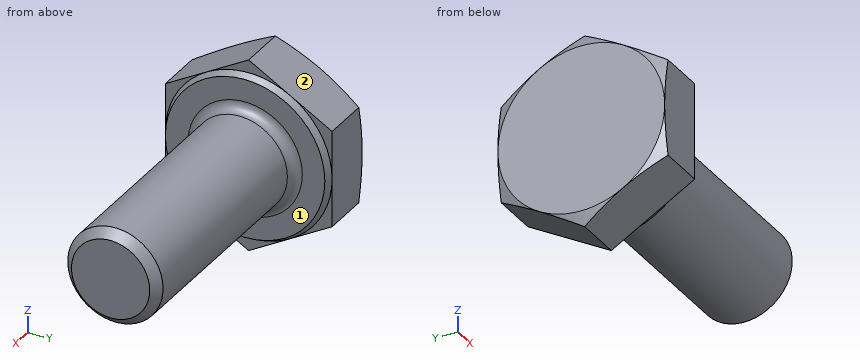
Autodesk Inventor part; units mm, degrees
ref_plane "Work Plane1" through (0, 10.5, -6.0622) normal (0, 0.5, 0.8660254) x (-1, 0, 0)
ref_plane "YZ Plane" through (0, 0, 0) normal (1, 0, 0) x (0, 1, 0)
ref_plane "XZ Plane" through (0, 0, 0) normal (0, 1, 0) x (-1, 0, 0)
sketch "草图4" plane through (0, 0, 0) normal (0, 0, 1) x (1, 0, 0)
  line L0 (0, 0) -> (0, 10.5)
  line L1 (0, 10.5) -> (0.8, 10.0381)
  line L2 (0.8, 10.0381) -> (0.8, 0)
  line L3 (0.8, 0) -> (0, 0)
  line L4 (0, 0) -> (10.723, 0)
  line L5 (0.8, 0) -> (30.8, 0)
  line L6 (30.8, 0) -> (30.8, 6)
  line L7 (30.8, 6) -> (0.8, 6)
  line L8 (0.8, 6) -> (0.8, 0)
  dimension "INC" = 0.8
  dimension "d22" = 60
  dimension "L" = 30
  dimension "D" = 12
  dimension "INS" = 21
revolve "Revolution3" add sketch "草图4" angle 360 about axis through (0, 0, 0) along (1, 0, 0)
sketch "草图5" plane through (0, 0, 0) normal (-1, 0, 0) x (0, 0, 1)
  line L0 (-6.0622, 10.5) -> (6.0622, 10.5)
  line L1 (6.0622, 10.5) -> (12.1244, 0)
  line L2 (12.1244, 0) -> (6.0622, -10.5)
  line L3 (6.0622, -10.5) -> (-6.0622, -10.5)
  line L4 (-6.0622, -10.5) -> (-12.1244, 0)
  line L5 (-12.1244, 0) -> (-6.0622, 10.5)
  point P0 (0, 0)
  point P1 (0, 0)
  dimension "d27" = 21
extrude "Extrusion2" add sketch "草图5" along normal blind 6.7
ref_plane "Work Plane1" through (0, 10.5, -6.0622) normal (0, 0.5, 0.8660254) x (-1, 0, 0)
sketch "草图6" plane through (0, 10.5, -6.0622) normal (0, 0.5, 0.8660254) x (-1, 0, 0)
  line L0 (0, 12.1244) -> (11.8845, 12.1244) construction
  line L1 (6.7, 6.0622) -> (6.7, 0)
  line L2 (0, 3.0311) -> (0, 0)
  line L3 (6.7, 6.0622) -> (6.7, 0)
  line L4 (0, 0) -> (6.7, 0)
  line L5 (0, 3.0311) -> (0, 0)
  line L6 (0, 6.0622) -> (0, 3.0311)
  line L7 (0, 6.0622) -> (6.7, 6.0622)
  line L8 (6.7, 1.6244) -> (5.9426, 0)
  dimension "d30" = 25
  dimension "d31" = 21
revolve "Revolution4" cut sketch "草图6" angle 360 about axis through (0, 0, 0) along (-1, 0, 0) contours L1 L4 L8
thread "Thread2"
chamfer "Chamfer2" distance 1.0735 angle 45 1 edges at (30.8, -6, 0)
fillet "Fillet1" radius 1.2 1 edges at (0.8, -6, 0)
equation "\"d27\" = INS"
equation "\"d28\" = KOH - INC"
equation "\"d33\" = NLG - LS"
equation "\"d35\" = GUL"
equation "\"L\" = NLG"
equation "\"D\" = NND"
equation "\"d31\" = INS"
equation "\"NND\" = 12"
equation "\"NLG\" = 30"
equation "\"PTC\" = 1.75"
equation "\"KOD\" = 1"
equation "\"KOH\" = 7.5"
equation "\"GUL\" = 0.61345 * PTC"
equation "\"LS\" = 0"
properties part number "Bolt GB/T 18230.2-2000 M12 x 30" material "Steel, Mild"
Input: part model. Units: mm. Frame: model coordinates. Face numbers are marked on the shaded views. A direction names the side the tool comes from. Coordinates: 2 decimals unless noted, no trailing zeros. Loops run counter-clockwise (first coordinate to the right, second up) from the corner with the lowest first, then second, coordinate; pieces in that order, holes last.
Q1. Set-up query: the marked faces 1 and 2. Return all of +Z, -Z, +X, -X, +Y, -Y with unobstructed straight access to the full face (end or side cutting, diameter ignored); none if empty.
Q2. Material intervals for line 1 (X direction, y = 9.25, z = -2); line 2 (Z direction, x = 4.5, y = -0.25); line 3 (Z direction, x = 13, y = -4.75), sorted ascending.
Q3. Cut plane A-A (x = 5). Output: boundary loops of the cut face in (y, z), then the cut area to 3 significant figures.
Q4. Contact query for flat-ended pins moving along their axis: pin 1 (4 mm diameter, centred on y = -7.5, z = -5, fed in from +X); pin 2 (3 mm diameter, centred on x = 2.5, y = -6, fed in from -Z); pin 3 (4 mm diameter, centred on y = 8, z = 3, fed in from +X). Output: stop coordinate, or through.
Working result:
1. face 1: +X
1. face 2: +Z, +X, -X, +Y
2. line 1: x = -6.7 to 0.8
2. line 2: z = -5.99 to 5.99
2. line 3: z = -3.67 to 3.67
3. outline: circle Ø12 at (0, 0)
3. area: 113 mm2
4. pin 1: stops at x = 0.81
4. pin 2: stops at z = -3.97
4. pin 3: stops at x = 1
